The model under review builds one solid part; all positions refer to its coordinate system, in mm. Face numbers are marked on the shaded views. A direction names the side the tool comes from. Round coordinates to 2 decimals unless told otherwise and drop trailing zeros. Loops run counter-clockwise (first coordinate to the right, second up) from the corner with the lowest first, then second, coordinate; pieces in that order, holes last. Notation, with made-up numbers: (-15.5, 66.5) - (7.5, 66.5) arc R11 cw to (7.5, 75.5) - close; hole circle Ø2 at (29, -34.5). An arc over 180 degrees is marked (long way). Answer as CSV lines item,"result".
from build123d import *

# Parameters (mm, degrees)
F1_DEPTH  = 6.2
F3_DEPTH  = 6.2
F5_DEPTH  = 10
F6_W      = 50
F6_H      = 50
F6_R      = 19
F7_DEPTH  = 6.2
F9_DEPTH  = 10
F11_DEPTH = 6.2
F13_DEPTH = 10
F15_DEPTH = 6.2
F16_R     = 22.25
F17_DEPTH = 13
F19_D     = 35
F19_DEPTH = 35
F19_TIP   = 10.515060833


with BuildPart() as f1:
    # F0 (on Top) → F1 (new body)
    with BuildSketch(Plane.XY):
        with BuildLine():
            Line((102, 19), (11.0905365064, 19))
            ThreePointArc((11.0905365064, 19), (0, 22), (-11.0905365064, 19))
            Line((-11.0905365064, 19), (-19, 19))
            Line((-19, 19), (-102, -7))
            Line((-102, -7), (-102, -19))
            Line((-102, -19), (-11.0905365064, -19))
            ThreePointArc((-11.0905365064, -19), (0, -22), (11.0905365064, -19))
            Line((11.0905365064, -19), (19, -19))
            Line((19, -19), (102, 7))
            Line((102, 7), (102, 19))
        make_face()
    extrude(amount=F1_DEPTH)

    # F2 (on face) → F3 (join)
    with BuildSketch(Plane(origin=(0, 0, 0), x_dir=(1, 0, 0), z_dir=(0, 0, -1))):
        with BuildLine():
            Line((-19, 19), (-19, 0))
            Line((-19, 0), (-19, -19))
            Line((-19, -19), (-11.0905365064, -19))
            ThreePointArc((-11.0905365064, -19), (0, -22), (11.0905365064, -19))
            Line((11.0905365064, -19), (19, -19))
            Line((19, -19), (19, 0))
            Line((19, 0), (19, 19))
            Line((19, 19), (11.0905365064, 19))
            ThreePointArc((11.0905365064, 19), (0, 22), (-11.0905365064, 19))
            Line((-11.0905365064, 19), (-19, 19))
        make_face()
        with BuildLine():
            Line((-11.0905365064, -19), (-19, -19))
            Line((-19, -19), (-19, -102))
            Line((-19, -102), (-7, -102))
            Line((-7, -102), (19, -19))
            Line((19, -19), (11.0905365064, -19))
            ThreePointArc((11.0905365064, -19), (0, -22), (-11.0905365064, -19))
        make_face()
        with BuildLine():
            Line((7, 102), (-19, 19))
            Line((-19, 19), (-11.0905365064, 19))
            ThreePointArc((-11.0905365064, 19), (0, 22), (11.0905365064, 19))
            Line((11.0905365064, 19), (19, 19))
            Line((19, 19), (19, 102))
            Line((19, 102), (7, 102))
        make_face()
    extrude(amount=F3_DEPTH)

    # F4 (on face) → F5 (join)
    with BuildSketch(Plane(origin=(0, 0, -6.2), x_dir=(1, 0, 0), z_dir=(0, 0, -1))):
        with BuildLine():
            ThreePointArc((-19, 0), (0, -19), (19, 0))
            ThreePointArc((19, 0), (0, 19), (-19, 0))
        make_face()
    extrude(amount=F5_DEPTH)

    # F6 (on face) → F7 (join)
    with BuildSketch(Plane(origin=(0, 0, -16.2), x_dir=(1, 0, 0), z_dir=(0, 0, -1))):
        Rectangle(F6_W, F6_H)
        Circle(F6_R, mode=Mode.SUBTRACT)
        Polygon((25, 25), (25, -25), (88, -25), (88, -13), align=None)
        Polygon((-88, 13), (-25, -25), (-25, 25), (-88, 25), align=None)
        Circle(F6_R)
    extrude(amount=F7_DEPTH)

    # F8 (on face) → F9 (join)
    with BuildSketch(Plane(origin=(0, 0, -22.4), x_dir=(1, 0, 0), z_dir=(0, 0, -1))):
        with BuildLine():
            ThreePointArc((-5.83e-08, -25), (17.677669509, -17.6776695503), (25, 0))
            ThreePointArc((25, 0), (17.6776695297, 17.6776695297), (0, 25))
            ThreePointArc((0, 25), (-25, 2.92e-08), (-5.83e-08, -25))
        make_face()
    extrude(amount=F9_DEPTH)

    # F10 (on face) → F11 (join)
    with BuildSketch(Plane(origin=(0, 0, -32.4), x_dir=(1, 0, 0), z_dir=(0, 0, -1))):
        Polygon((13, 75), (-25, 25), (4.22e-08, 25), (25, 25), (25, 75), align=None)
        with BuildLine():
            ThreePointArc((4.22e-08, 25), (17.6776695446, 17.6776695147), (25, 0))
            Line((25, 0), (25, 25))
            Line((25, 25), (4.22e-08, 25))
        make_face()
        with BuildLine():
            ThreePointArc((-25, 0), (-17.6776695332, -17.6776695262), (-9.9e-09, -25))
            ThreePointArc((-9.9e-09, -25), (17.6776695262, -17.6776695332), (25, 0))
            ThreePointArc((25, 0), (17.6776695446, 17.6776695147), (4.22e-08, 25))
            ThreePointArc((4.22e-08, 25), (-17.6776695147, 17.6776695446), (-25, 0))
        make_face()
        with BuildLine():
            ThreePointArc((25, 0), (17.6776695262, -17.6776695332), (-9.9e-09, -25))
            Line((-9.9e-09, -25), (25, -25))
            Line((25, -25), (25, 0))
        make_face()
        Polygon((-9.9e-09, -25), (-25, -25), (-25, -75), (-13, -75), (25, -25), align=None)
        with BuildLine():
            Line((-25, 0), (-25, -25))
            Line((-25, -25), (-9.9e-09, -25))
            ThreePointArc((-9.9e-09, -25), (-17.6776695332, -17.6776695262), (-25, 0))
        make_face()
        with BuildLine():
            Line((-25, 25), (-25, 0))
            ThreePointArc((-25, 0), (-17.6776695147, 17.6776695446), (4.22e-08, 25))
            Line((4.22e-08, 25), (-25, 25))
        make_face()
    extrude(amount=F11_DEPTH)

    # F12 (on face) → F13 (join)
    with BuildSketch(Plane(origin=(0, 0, -38.6), x_dir=(1, 0, 0), z_dir=(0, 0, -1))):
        with BuildLine():
            ThreePointArc((-25, 2.61e-08), (-1.3e-08, -25), (25, 0))
            ThreePointArc((25, 0), (1.3e-08, 25), (-25, 2.61e-08))
        make_face()
    extrude(amount=F13_DEPTH)

    # F14 (on face) → F15 (join)
    with BuildSketch(Plane(origin=(0, 0, -48.6), x_dir=(1, 0, 0), z_dir=(0, 0, -1))):
        with BuildLine():
            ThreePointArc((-25, 0), (-17.6776695204, -17.6776695389), (2.61e-08, -25))
            ThreePointArc((2.61e-08, -25), (17.6776695389, -17.6776695204), (25, 0))
            ThreePointArc((25, 0), (17.6776695389, 17.6776695204), (2.61e-08, 25))
            ThreePointArc((2.61e-08, 25), (-17.6776695204, 17.6776695389), (-25, 0))
        make_face()
        with BuildLine():
            ThreePointArc((2.61e-08, 25), (17.6776695389, 17.6776695204), (25, 0))
            Line((25, 0), (25, 25))
            Line((25, 25), (2.61e-08, 25))
        make_face()
        with BuildLine():
            Line((2.61e-08, -25), (25, -25))
            Line((25, -25), (25, 0))
            ThreePointArc((25, 0), (17.6776695389, -17.6776695204), (2.61e-08, -25))
        make_face()
        with BuildLine():
            Line((-25, -25), (2.61e-08, -25))
            ThreePointArc((2.61e-08, -25), (-17.6776695204, -17.6776695389), (-25, 0))
            Line((-25, 0), (-25, -25))
        make_face()
        with BuildLine():
            Line((-25, 25), (-25, 0))
            ThreePointArc((-25, 0), (-17.6776695204, 17.6776695389), (2.61e-08, 25))
            Line((2.61e-08, 25), (-25, 25))
        make_face()
        Polygon((-50, 13), (-25, -25), (-25, 0), (-25, 25), (-50, 25), align=None)
        Polygon((25, 0), (25, -25), (50, -25), (50, -13), (25, 25), align=None)
    extrude(amount=F15_DEPTH)

    # F16 (on face) → F17 (join)
    with BuildSketch(Plane(origin=(0, 0, -54.8), x_dir=(1, 0, 0), z_dir=(0, 0, -1))):
        Circle(F16_R)
    extrude(amount=F17_DEPTH)

    # F19
    with Locations(Plane(origin=(0, 0, -67.8), x_dir=(1, 0, 0), z_dir=(0, 0, -1))):
        with Locations((0, 0)):
            Hole(F19_D / 2, depth=F19_DEPTH)
            with Locations((0, 0, -(F19_DEPTH + F19_TIP / 2))):  # 118° drill point
                Cone(0, F19_D / 2, F19_TIP, mode=Mode.SUBTRACT)


solid = f1.part
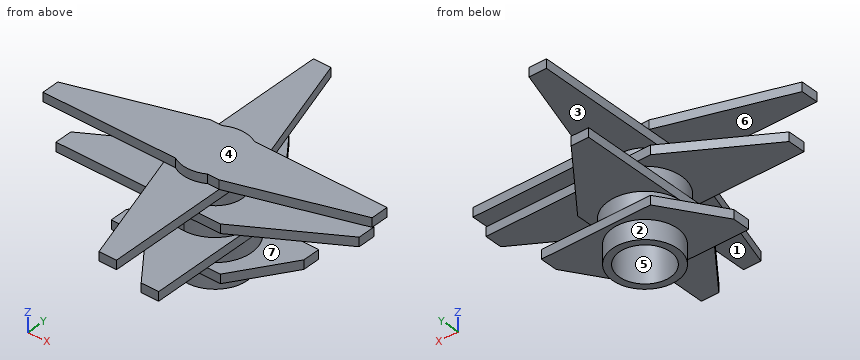
1. Take a section at B-B (y = -72.5). State the section outline as (x, z) points, plus the area to 3 significant figures.
Numbers:
outline,"(-2.24, -6.2) - (19, -6.2) - (19, 0) - (-2.24, 0) - close; (11.1, -38.6) - (25, -38.6) - (25, -32.4) - (11.1, -32.4) - close"
area,"218 mm²"
2. Wall thickness on probe 1 along Z at (x, y) = (-31, -20); probe 2 along Y at (x, z) = (0, -40.5); probe 3 along Y at (x, z) = (-4.5, -22): over which ranges is each line inside the solid? List them lowest first.
Numbers:
probe 1,"z = -54.8 to -48.6, -22.4 to -16.2"
probe 2,"y = -25 to -17.5, 17.5 to 25"
probe 3,"y = -25 to 25"
3. Clearance check with flat-ended pins moving along their axes: pin 1 (5 mm diameter, centred on x = 29.5, z = -53, fed in from +Y); pin 2 (7 mm diameter, centred on y = -22, z = -20.5, fed in from -X); pin 3 (7 mm diameter, centred on y = 18, z = -19, fed in from +X). State where each tip first meets the part, or that it passes through.
Numbers:
pin 1,"stops at y = 25"
pin 2,"stops at x = -88"
pin 3,"stops at x = 88"
4. Take a section at A-A (x = 77). State the section outline as (y, z) points.
Numbers:
outline,"(-0.83, 0) - (19, 0) - (19, 6.2) - (-0.83, 6.2) - close; (6.37, -22.4) - (25, -22.4) - (25, -16.2) - (6.37, -16.2) - close"
5. Tool access review of the marked faces 5, 6 and 7: name each direction out of +Z, -Z, +X, -X, +Y, -Y from which nothing blocks a thin tool from reaching the whole face with its end or side.
Numbers:
face 5,"-Z"
face 6,"-X, +Y, -Y"
face 7,"+X"
6. Take a section at D-D (z = -30). State the section outline as (x, y) points, plus the area to 3 significant figures.
Numbers:
outline,"circle Ø50 at (0, 0); hole circle Ø25.68 at (0, 0)"
area,"1,450 mm²"
7. Draft analysis for pull direction Z (two halves, no side actions). For the marked faces 1, 2, 3 and 4, state which applies: +Z half, -Z half, draft (parallel to the pull), parting line (faces both ways), or undercut.
Numbers:
face 1,"undercut"
face 2,"draft"
face 3,"undercut"
face 4,"+Z half"
8. Take a section at C-C (x = 31). State the section outline as (y, z) points.
Numbers:
outline,"(-21.38, -22.4) - (25, -22.4) - (25, -16.2) - (-21.38, -16.2) - close; (-15.88, -54.8) - (25, -54.8) - (25, -48.6) - (-15.88, -48.6) - close; (-15.24, 0) - (19, 0) - (19, 6.2) - (-15.24, 6.2) - close"
